Can you work these out from the model? Positions are in its coordinate system, mm. A direction names the side the tool comes from. Give positions to 0.01 mm unless a question says otherwise; leave off trailing zeros. Loops run counter-clockwise (first coordinate to the right, second up) from the corner with the lowest first, then second, coordinate; pieces in that order, holes last. Notation, with made-up numbers: M 6.5,7 L 54.5,7 A35 ccw 54.5,39 Z; hole C 24.5,25.25 d8. An arc over 180 degrees is marked long. Answer as a JSON object with one key per item and string values.
```python
from build123d import *

# Parameters (mm, degrees)
SKETCH1_W           = 75
SKETCH1_H           = 50
BOSS_EXTRUDE1_DEPTH = 150
SKETCH2_R           = 2.369647205
BOSS_EXTRUDE2_DEPTH = 10
BOSS_EXTRUDE3_START = 10
SKETCH3_R           = 2.369647205
BOSS_EXTRUDE3_DEPTH = 10


with BuildPart() as part:
    # Sketch1 → Boss-Extrude1 (new body)
    with BuildSketch(Plane.XY):
        Rectangle(SKETCH1_W, SKETCH1_H)
    extrude(amount=BOSS_EXTRUDE1_DEPTH)

    # Sketch2 → Boss-Extrude2 (add)
    with BuildSketch(Plane(origin=(37.5, 0, 0), x_dir=(0, 0, -1), z_dir=(1, 0, 0))):
        with Locations(Location((-125, -16.919154578, 0), (0, 0, 270))):
            Circle(SKETCH2_R)
        with Locations(Location((-25, -16.919154578, 0), (0, 0, 270))):
            Circle(SKETCH2_R)
    extrude(amount=BOSS_EXTRUDE2_DEPTH)

    # Sketch3 → Boss-Extrude3 (add)
    with BuildSketch(Plane.ZY.offset(37.5).offset(BOSS_EXTRUDE3_START)):
        with Locations(Location((25, -16.919154578, 0), (0, 0, 270))):
            Circle(SKETCH3_R)
        with Locations(Location((125, -16.919154578, 0), (0, 0, 270))):
            Circle(SKETCH3_R)
    extrude(amount=-BOSS_EXTRUDE3_DEPTH)


solid = part.part
```
1) Will these pins go through, and if not, where does the flat tip stop? pin 1 Ø1 at (y, z) = (-4.5, 52) entering from -X; pin 2 Ø3 at (x, y) = (0, -18) entering from -Z; pin 3 Ø4 at (y, z) = (-9.5, 28.5) entering from +X.
Answer list:
{"pin 1": "x = -37.5", "pin 2": "z = 0", "pin 3": "x = 37.5"}
2) Suppose I cut it at D-D, the plane z = 80. Write out the boundary of the cut face in (x, y).
Answer list:
{"outline": "M -37.5,-25 L 37.5,-25 L 37.5,25 L -37.5,25 Z"}
3) Suppose I cut it at B-B, the plane x = 41.5. Write out the boundary of the cut face in (y, z), and give its area (3 significant figures).
Answer list:
{"outline": "C -16.92,25 d4.74; C -16.92,125 d4.74", "area": "35.3 mm^2"}
4) Suppose I cut it at C-C, the plane y = 8. Write out the boundary of the cut face in (x, z), and give its area (4 significant figures).
Answer list:
{"outline": "M -37.5,0 L 37.5,0 L 37.5,150 L -37.5,150 Z", "area": "11,250 mm^2"}
5) Suppose I cut it at A-A, the plane z = 125. Write out the boundary of the cut face in (x, y).
Answer list:
{"outline": "M -47.5,-19.29 L -37.5,-19.29 L -37.5,-25 L 37.5,-25 L 37.5,-19.29 L 47.5,-19.29 L 47.5,-14.55 L 37.5,-14.55 L 37.5,25 L -37.5,25 L -37.5,-14.55 L -47.5,-14.55 Z"}
6) For faces 1 (the flat face through (-1, 25, 74)), 2 (the cylindrical face through (42.43, -16.405, 27.313)), 3 (the cylindrical face through (-42.57, -18.19, 127)), which set-ups out of +Z, -Z, +X, -X, +Y, -Y let a thin tool reach every point of the face, with its end or its side?
Answer list:
{"face 1": "+Z, -Z, +X, -X, +Y", "face 2": "+X", "face 3": "-X"}
7) Please list where these lines run through material, in increasing order: line 1 along X through (y, z) = (20.5, 75); line 2 along Z through (x, y) = (42, -15). Write a range as from..to.
Answer list:
{"line 1": "-37.5..37.5", "line 2": "23.61..26.39, 123.61..126.39"}
8) If we mould it in two halves opening along Z, with no side actions, what happens to faces 4 (the cylindrical face through (-42.57, -16.405, 22.687)), 5 (the cylindrical face through (42.43, -18.19, 123)), 6 (the flat face through (-1, 0, 0)), 7 (the flat face through (47.5, -17, 125))? For each: +Z half, -Z half, draft (parallel to the pull), parting line (faces both ways), or undercut.
Answer list:
{"face 4": "undercut", "face 5": "undercut", "face 6": "-Z half", "face 7": "draft"}
